Here's how the part is built. I have some questions about the finished solid (model axes, mm). Face numbers are marked on the shaded views. A direction names the side the tool comes from. Round coordinates to 2 decimals unless told otherwise and drop trailing zeros. Write each loop counter-clockwise with the first axis right and the second up, starting at its lowest first coordinate (ties: lowest second). Pieces come first, ordered by that corner, then holes. Notation, with made-up numbers: M 55,59 L 63,59 A12 cw 63,73 Z; hole C -35,85 d2. An arc over 180 degrees is marked long. Write item = value, one per line. Start each with the question number.
(1) I want a section at D-D (y = 4.25). List the corners of the cut face in (x, z) for me, and give its area (3 significant figures).
(2) Will these pins go through, and if not, where does the flat tip stop? pin 1 Ø1.2 at (x, z) = (-1, -1) entering from +Y; pin 2 Ø1.5 at (y, z) = (-7, 0.5) entering from +X; pin 3 Ø1 at (y, z) = (-5.5, 1) entering from +X.
(3) On a 3-axis mill with a long thin cutter (end or side, diameter ignored), from which of +Z, -Z, +X, -X, +Y, -Y can I reach the whole of each face in a straight line? I mean the marked faces 4 and 5. Say none if no direction works.
(4) I want a section at C-C (y = 1.5). List the corners of the cut face in (x, z) for me, and give its area (3 significant figures).
(5) I want a section at A-A (x = 0). List the corners of the cut face in (y, z) for me.
(6) I want a section at B-B (z = -0.75). List the corners of the cut face in (x, y) for me.
(7) I need wall thicknesses on line 1 along Y through (x, z) = (0, -3.5); line 2 along Z through (x, y) = (-3, 4); line 3 along Y through (x, z) = (4, -2). Which ranges of each line are inside material? Lowest first, please.
(8) If we mould it in two halves opening along Y, with no side actions, what happens to the marked faces 1, 2 and 3? For each: released by +Y, released by -Y, zero draft, split by the parting line, or undercut.
Autodesk Fusion 360 part; units mm, degrees
sketch "Sketch1" plane through (0, 0, 0) normal (0, 0, 1) x (1, 0, 0)
  circle A0 centre (0, 0) radius 9
  circle A1 centre (0, 0) radius 6 construction
  circle A2 centre (-0.0008, 6) radius 2
  circle A3 centre (-6, -0.0008) radius 2
  circle A4 centre (0.0008, -6) radius 2
  circle A5 centre (6, 0.0008) radius 2
  circle A6 centre (0, 0) radius 2.1
  dimension "d1" = 18
  dimension "d2" = 12
  dimension "d3" = 4
  dimension "d5" = 360
  dimension "d25" = 4.2
extrude "Extrude1" add sketch "Sketch1" against normal blind 4 contours A0 | A2 | A3 | A4 | A5
extrude "Extrude2" add sketch "Sketch1" along normal blind 3 contours A2 | A3 | A4 | A5
sketch "Sketch7" plane through (0, 0, 0) normal (0, 0, 1) x (-1, 0, 0)
  circle A0 centre (-6, -0.0008) radius 2
  circle A1 centre (6, 0.0008) radius 2
  circle A2 centre (0.0008, -6) radius 2
  circle A3 centre (-0.0008, 6) radius 2
  circle A4 centre (0, 0) radius 2.1
  circle A5 centre (0, 0) radius 9
  line L0 (-4.1569, 0) -> (-2.0785, -3.6)
  line L1 (-2.0785, -3.6) -> (2.0785, -3.6)
  line L2 (2.0785, -3.6) -> (4.1569, 0)
  line L3 (4.1569, 0) -> (2.0785, 3.6)
  line L4 (2.0785, 3.6) -> (-2.0785, 3.6)
  line L5 (-2.0785, 3.6) -> (-4.1569, 0)
  dimension "d26" = 7.2
extrude "Extrude8" cut sketch "Sketch7" against normal blind 2.5 contours A0 L0 L5 | A0 A1 L0 L1 L2 L3 L4 L5 | A1 L2 L3 picked at (-4.0529, 0.0269) picked at (4.0534, 0.0001)
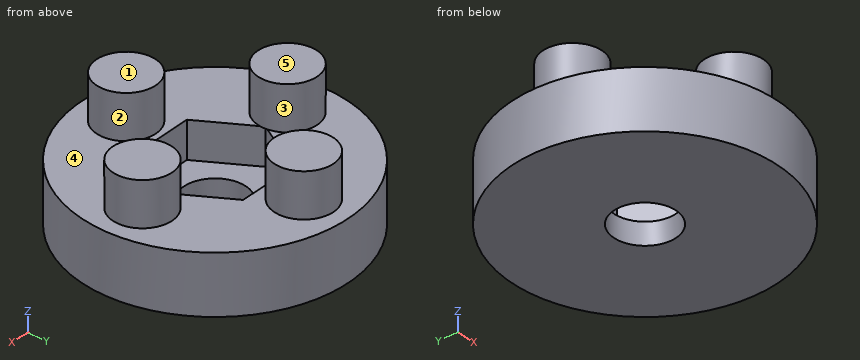
Returned:
q1.outline = M -7.93,-4 L 7.93,-4 L 7.93,0 L 0.97,0 L 0.97,3 L -0.97,3 L -0.97,0 L -7.93,0 Z
q1.area = 69.3 mm²
q2.pin_1 = 8.99
q2.pin_2 = 6.29
q2.pin_3 = 2
q3.face_4 = +Z
q3.face_5 = +Z, +X, -X, +Y, -Y
q4.outline = M -8.87,-4 L -1.47,-4 L -1.47,-2.5 L -3.29,-2.5 L -3.29,0 L -4.68,0 L -4.68,3 L -7.32,3 L -7.32,0 L -8.87,0 Z; M 1.47,-4 L 8.87,-4 L 8.87,0 L 7.32,0 L 7.32,3 L 4.68,3 L 4.68,0 L 3.29,0 L 3.29,-2.5 L 1.47,-2.5 Z
q4.area = 66.0 mm²
q5.outline = M -9,-4 L -2.1,-4 L -2.1,-2.5 L -3.6,-2.5 L -3.6,0 L -4,0 L -4,3 L -8,3 L -8,0 L -9,0 Z; M 2.1,-4 L 9,-4 L 9,0 L 8,0 L 8,3 L 4,3 L 4,0 L 3.6,0 L 3.6,-2.5 L 2.1,-2.5 Z
q6.outline = C 0,0 d18; hole M -4.16,0 L -2.08,-3.6 L 2.08,-3.6 L 4.16,0 L 2.08,3.6 L -2.08,3.6 Z
q7.line_1 = -9 to -2.1, 2.1 to 9
q7.line_2 = -4 to 0
q7.line_3 = -8.06 to -0.27, 0.27 to 8.06
q8.face_1 = zero draft
q8.face_2 = undercut
q8.face_3 = split by the parting line
